from build123d import *

# Parameters (mm, degrees)
SKETCH1_W           = 142.24
SKETCH1_H           = 60.325
BOSS_EXTRUDE1_DEPTH = 6.35
SKETCH2_R           = 2
SKETCH2_W           = 6.35
SKETCH2_H           = 12.7
CUT_EXTRUDE1_DEPTH  = 155.633908717
SKETCH3_W           = 12.7
SKETCH3_H           = 6.35
BOSS_EXTRUDE2_DEPTH = 6.35


with BuildPart() as part:
    # Sketch1 → Boss-Extrude1 (new body)
    with BuildSketch(Plane(origin=(0, 0, 0), x_dir=(1, 0, 0), z_dir=(0, 1, 0))):
        with Locations((71.12, -30.1625)):
            Rectangle(SKETCH1_W, SKETCH1_H)
    extrude(amount=BOSS_EXTRUDE1_DEPTH)

    # Sketch2 → Cut-Extrude1 (cut, through all)
    with BuildSketch(Plane(origin=(0, 6.35, 0), x_dir=(1, 0, 0), z_dir=(0, 1, 0))):
        with Locations(Location((6.35, -15.225, 0), (0, 0, 270))):
            Circle(SKETCH2_R)
        with Locations(Location((6.35, -45.225, 0), (0, 0, 270))):
            Circle(SKETCH2_R)
        with Locations(Location((135.89, -45.225, 0), (0, 0, 90))):
            Circle(SKETCH2_R)
        with Locations(Location((135.89, -15.225, 0), (0, 0, 90))):
            Circle(SKETCH2_R)
        with Locations((126.365, -30.1625)):
            Rectangle(SKETCH2_W, SKETCH2_H)
        with Locations((15.875, -30.1625)):
            Rectangle(SKETCH2_W, SKETCH2_H)
    extrude(amount=-CUT_EXTRUDE1_DEPTH, mode=Mode.SUBTRACT)

    # Sketch3 → Boss-Extrude2 (add)
    with BuildSketch(Plane(origin=(0, 6.35, 0), x_dir=(1, 0, 0), z_dir=(0, 1, 0))):
        with Locations((25.4, 3.175)):
            Rectangle(SKETCH3_W, SKETCH3_H)
        with Locations((116.84, 3.175)):
            Rectangle(SKETCH3_W, SKETCH3_H)
        with Locations((116.84, -63.5)):
            Rectangle(SKETCH3_W, SKETCH3_H)
        with Locations((25.4, -63.5)):
            Rectangle(SKETCH3_W, SKETCH3_H)
        with Locations((71.12, -63.5)):
            Rectangle(SKETCH3_W, SKETCH3_H)
        with Locations((71.12, 3.175)):
            Rectangle(SKETCH3_W, SKETCH3_H)
    extrude(amount=-BOSS_EXTRUDE2_DEPTH)


solid = part.part
Read the model definition and answer for the solid it produces. Units are mm, in the model's axes. A direction names the side the tool comes from. Coordinates: 2 decimals unless noted, no trailing zeros. Order: outer loops, then holes, each group sorted by start corner. A loop starts at its lowest first (then second) coordinate and runs counter-clockwise, first axis right, second up. Notation, with made-up numbers: M 7,60.25 L 57,60.25 A27 ccw 57,86.25 Z; hole C 87.25,-12.5 d3. An arc over 180 degrees is marked long. Put each result on its own line as item: value. Start each with the question number.
Item 1: For faces 4 (the face through (123.19, 3, -3)), 5 (the face through (110.49, 3, -3)), 6 (the face through (64.77, 3, 64)), determine the directions among +Z, -Z, +X, -X, +Y, -Y from which every point of the face is accessible in a straight line to the end or side of a thin tool.
Item 2: Consider probe 1 along Z at (x, y) = (135.89, 3) (3 decimals); probe 2 along X at (y, z) = (5.25, -1); probe 3 along X at (y, z) = (4.25, 32.5). Determine where each line is inside the solid, lowest interval first. Write a range as [from, to].
Item 3: Section B-B, the plane x = 135.89 is taken. Determine the outline of the cut face in (y, z) (3 decimals).
Item 4: Section A-A, the plane z = 62 is taken. Determine the outline of the cut face in (x, y).
Item 5: Section C-C, the plane y = 2 is taken. Count the separate pieces of the cut face and the enclosed holes in it, plus the area to 3 significant figures.
Item 6: Given pin 1 Ø1.9 at (x, y) = (127.5, 2.5) entering from +Z (3 decimals); pin 2 Ø1.9 at (y, z) = (2, 65) entering from -X; pin 3 Ø3 at (y, z) = (2, 65) entering from +X, each flat-ended and moving along its own axis, determine where each tip first touches the part or whether it passes through.
Item 7: The mould has two halves that part along X. Classify faces 1 (the face through (123.19, 3, 30)), 2 (the face through (123.19, 3, 64)), 3 (the face through (9, 3, 0)): +X half, -X half, draft (parallel to the pull), parting line (faces both ways), or undercut.
Computed:
1. face 4: -Z, +X, +Y, -Y
1. face 5: -Z, +Y, -Y
1. face 6: +Z, +Y, -Y
2. probe 1: z = [0, 13.225], [17.225, 43.225], [47.225, 60.325]
2. probe 2: x = [19.05, 31.75], [64.77, 77.47], [110.49, 123.19]
2. probe 3: x = [0, 12.7], [19.05, 123.19], [129.54, 142.24]
3. outline: M 0,0 L 6.35,0 L 6.35,13.225 L 0,13.225 Z; M 0,17.225 L 6.35,17.225 L 6.35,43.225 L 0,43.225 Z; M 0,47.225 L 6.35,47.225 L 6.35,60.325 L 0,60.325 Z
4. outline: M 19.05,0 L 31.75,0 L 31.75,6.35 L 19.05,6.35 Z; M 64.77,0 L 77.47,0 L 77.47,6.35 L 64.77,6.35 Z; M 110.49,0 L 123.19,0 L 123.19,6.35 L 110.49,6.35 Z
5. separate pieces: 1
5. enclosed holes: 6
5. area: 8,850 mm2
6. pin 1: stops at z = 60.325
6. pin 2: stops at x = 19.05
6. pin 3: stops at x = 123.19
7. face 1: undercut
7. face 2: +X half
7. face 3: draft
